from build123d import *

# Parameters (mm, degrees)
ESQUISSE2_W        = 82
ESQUISSE2_H        = 22
ESQUISSE2_R        = 4.05
ESQUISSE2_R_2      = 1
BOSS_EXTRU_1_DEPTH = 2
CONG_1_R           = 10


with BuildPart() as part:
    # Esquisse2 → Boss.-Extru.1 (new body)
    with BuildSketch(Plane(origin=(0, 0, 0), x_dir=(-1, 0, 0), z_dir=(0, 0, -1))):
        with Locations((-41, 0)):
            Rectangle(ESQUISSE2_W, ESQUISSE2_H)
        with Locations((-11, 0)):
            Circle(ESQUISSE2_R, mode=Mode.SUBTRACT)
        with Locations((-4, 0)):
            Circle(ESQUISSE2_R_2, mode=Mode.SUBTRACT)
        with Locations((-4.937822174, -3.5)):
            Circle(ESQUISSE2_R_2, mode=Mode.SUBTRACT)
        with Locations((-7.5, -6.062177826)):
            Circle(ESQUISSE2_R_2, mode=Mode.SUBTRACT)
        with Locations((-11, -7)):
            Circle(ESQUISSE2_R_2, mode=Mode.SUBTRACT)
        with Locations((-14.5, -6.062177826)):
            Circle(ESQUISSE2_R_2, mode=Mode.SUBTRACT)
        with Locations((-17.062177826, -3.5)):
            Circle(ESQUISSE2_R_2, mode=Mode.SUBTRACT)
        with Locations((-18, 0)):
            Circle(ESQUISSE2_R_2, mode=Mode.SUBTRACT)
        with Locations((-17.062177826, 3.5)):
            Circle(ESQUISSE2_R_2, mode=Mode.SUBTRACT)
        with Locations((-14.5, 6.062177826)):
            Circle(ESQUISSE2_R_2, mode=Mode.SUBTRACT)
        with Locations((-11, 7)):
            Circle(ESQUISSE2_R_2, mode=Mode.SUBTRACT)
        with Locations((-7.5, 6.062177826)):
            Circle(ESQUISSE2_R_2, mode=Mode.SUBTRACT)
        with Locations((-4.937822174, 3.5)):
            Circle(ESQUISSE2_R_2, mode=Mode.SUBTRACT)
        with Locations((-71, 0)):
            Circle(ESQUISSE2_R, mode=Mode.SUBTRACT)
        with Locations((-64, 0)):
            Circle(ESQUISSE2_R_2, mode=Mode.SUBTRACT)
        with Locations((-64.937822174, -3.5)):
            Circle(ESQUISSE2_R_2, mode=Mode.SUBTRACT)
        with Locations((-67.5, -6.062177826)):
            Circle(ESQUISSE2_R_2, mode=Mode.SUBTRACT)
        with Locations((-71, -7)):
            Circle(ESQUISSE2_R_2, mode=Mode.SUBTRACT)
        with Locations((-74.5, -6.062177826)):
            Circle(ESQUISSE2_R_2, mode=Mode.SUBTRACT)
        with Locations((-77.062177826, -3.5)):
            Circle(ESQUISSE2_R_2, mode=Mode.SUBTRACT)
        with Locations((-78, 0)):
            Circle(ESQUISSE2_R_2, mode=Mode.SUBTRACT)
        with Locations((-77.062177826, 3.5)):
            Circle(ESQUISSE2_R_2, mode=Mode.SUBTRACT)
        with Locations((-74.5, 6.062177826)):
            Circle(ESQUISSE2_R_2, mode=Mode.SUBTRACT)
        with Locations((-71, 7)):
            Circle(ESQUISSE2_R_2, mode=Mode.SUBTRACT)
        with Locations((-67.5, 6.062177826)):
            Circle(ESQUISSE2_R_2, mode=Mode.SUBTRACT)
        with Locations((-64.937822174, 3.5)):
            Circle(ESQUISSE2_R_2, mode=Mode.SUBTRACT)
    extrude(amount=-BOSS_EXTRU_1_DEPTH)

    # Congé1
    cong_1_edges = [part.edges().sort_by_distance(p)[0] for p in [
        (82, 11, 1),
        (0, 11, 1),
        (0, -11, 1),
        (82, -11, 1),
    ]]
    fillet(cong_1_edges, radius=CONG_1_R)


solid = part.part
Read the model definition and answer for the solid it produces. Units are mm, in the model's axes. Coordinates: 2 decimals unless noted, no trailing zeros. Answer in a Markdown table with one row per item.
Q1. Find section A-A on z = 1.1. Count the separate pieces of the cut face and the enclosed holes in it, plus the area to 3 significant figures.
Here are the results:
| item | result |
|---|---|
| separate pieces | 1 |
| enclosed holes | 26 |
| area | 1,540 mm^2 |
Q2. The mould has two halves that part along Y. Classify faces 1 (the flat face through (41, -11, 1)), 2 (the cylindrical face through (65, 0, 1)), 3 (the flat face through (82, 0, 1)): pulls with the +Y half, pulls with the -Y half, needs draft (parallel to the pull), parting line crosses it, or undercut.
Here are the results:
| item | result |
|---|---|
| face 1 | pulls with the -Y half |
| face 2 | undercut |
| face 3 | needs draft |
Q3. Straight lines are drawn through the part: line 1 along Y through (x, z) = (11, 1.2); line 2 along X through (y, z) = (1.75, 1.2); line 3 along Y through (x, z) = (7.5, 1.25). For each, find the intervals that lie inside material, in ascending order. Write a range as [from, to].
Here are the results:
| item | result |
|---|---|
| line 1 | y = [-11, -8], [-6, -4.05], [4.05, 6], [8, 11] |
| line 2 | x = [0.03, 7.35], [14.65, 67.35], [74.65, 81.97] |
| line 3 | y = [-10.68, -7.06], [-5.06, -2.04], [2.04, 5.06], [7.06, 10.68] |
Q4. Given P1, Ø1.2, axis at x = 78, y = 0, coming from the -Z side; P2, Ø12, axis at x = 63.5, y = 8.5, coming from the -Z side, each flat-ended and moving along its own axis, determine where each tip first touches the part or whether it passes through.
Here are the results:
| item | result |
|---|---|
| P1 | passes through |
| P2 | stops at z = 0 |
